Part model, mm, in its own coordinate system. Face numbers are marked on the shaded views. A direction names the side the tool comes from. Give positions to 0.01 mm unless a question says otherwise; leave off trailing zeros. Write each loop counter-clockwise with the first axis right and the second up, starting at its lowest first coordinate (ties: lowest second). Pieces come first, ordered by that corner, then holes. Notation, with made-up numbers: M -16,14 L 18,14 A15 ccw 18,25 Z; hole C 80.25,73.5 d7. An arc over 180 degrees is marked long. Answer as CSV lines item,"result". Start each with the question number.
1) Tool access for the marked faces 4 and 5: list every direction of +Z, -Z, +X, -X, +Y, -Y with a clear straight run to the whole face (end or side of a thin tool).
2) Wall check: line 1 along X through (y, z) = (-7, 6.5); line 2 along Y through (x, z) = (8.5, 15.5); line 3 along Y through (x, z) = (37.5, 83). Give the ranges that are in metal, low to high. Write a range as from..to.
3) Slice it at C-C, the plane y = -46.5. Give the cut face in (x, z).
4) Slice it at B-B, the plane x = -1. Give the cut face in (y, z), plus the area to 3 significant figures.
5) Mould opens along X. For the marked faces 1, 2 and 3 say: pulls with the +X half, pulls with the -X half, needs draft (parallel to the pull), parting line crosses it, or undercut.
6) Pin check, flat tips, straight feed: pin 1 Ø12 at (x, y) = (24.5, 18) entering from -Z; pin 2 Ø2 at (x, z) = (-8, 82) entering from -Y. Stop position of each tip, or through.
7) Slice it at D-D, the plane x = -11.5. Give the cut face in (y, z), plus the area to 3 significant figures.
8) Slice it at A-A, the plane z = 17. Give the cut face in (x, y).
```python
from build123d import *

# Parameters (mm, degrees)
F0_W     = 76.2
F0_H     = 76.2
F1_DEPTH = 101.6
F3_DEPTH = 25.4
F5_D     = 20.32


with BuildPart() as f1:
    # F0 (on Top) → F1 (new body)
    with BuildSketch(Plane.XY):
        with Locations((2.984056, -3.896592)):
            Rectangle(F0_W, F0_H)
    extrude(amount=F1_DEPTH)

    # F2 (on face) → F3 (join)
    with BuildSketch(Plane.XZ.offset(41.996592)):
        Polygon((-35.115944, 38.1), (-35.115944, 0), (2.984056, 0), align=None)
    extrude(amount=F3_DEPTH)

    # F5 (through all)
    with Locations(Plane.XY.offset(101.6)):
        with Locations((2.984056, -3.896592)):
            Hole(F5_D / 2)


solid = f1.part
```
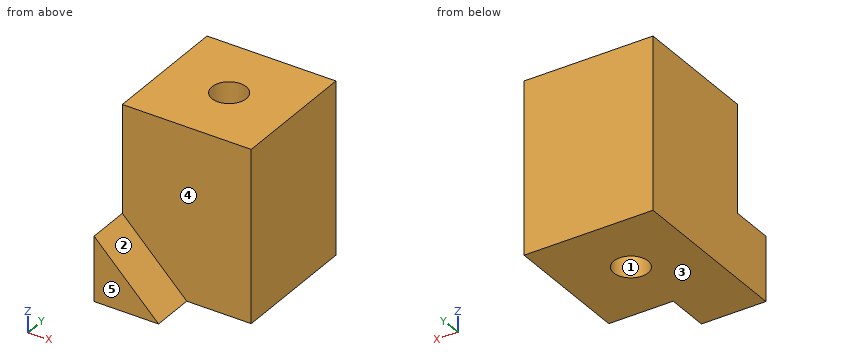
Found:
1,face 4,"+Z, +X, -Y"
1,face 5,"+Z, -Z, +X, -X, -Y"
2,line 1,"-35.12..-6.69, 12.66..41.08"
2,line 2,"-42..-12.43, 4.64..34.2"
2,line 3,"-42..34.2"
3,outline,"M -35.12,0 L 2.98,0 L -35.12,38.1 Z"
4,outline,"M -67.4,0 L -13.24,0 L -13.24,101.6 L -42,101.6 L -42,3.98 L -67.4,3.98 Z; M 5.45,0 L 34.2,0 L 34.2,101.6 L 5.45,101.6 Z"
4,area,"5,940 mm²"
5,face 1,"undercut"
5,face 2,"pulls with the +X half"
5,face 3,"needs draft"
6,pin 1,"z = 0"
6,pin 2,"y = -42"
7,outline,"M -67.4,0 L 34.2,0 L 34.2,101.6 L -42,101.6 L -42,14.48 L -67.4,14.48 Z"
7,area,"8,110 mm²"
8,outline,"M -35.12,-67.4 L -14.02,-67.4 L -14.02,-42 L 41.08,-42 L 41.08,34.2 L -35.12,34.2 Z; hole C 2.98,-3.9 d20.32"
